For this review, take the finished solid that the model builds, in its own axes (mm). Face numbers are marked on the shaded views. A direction names the side the tool comes from. Coordinates: 2 decimals unless noted, no trailing zeros. Loops run counter-clockwise (first coordinate to the right, second up) from the corner with the lowest first, then second, coordinate; pieces in that order, holes last. Notation, with made-up numbers: (-15.5, 24) - (-11.5, 24) arc R26 ccw to (-11.5, 42) - close; hole circle Ø3 at (-4.75, 76.25). An arc over 180 degrees is marked (long way). Answer as a JSON object with one key per item and string values. Group by question number.
Item 1: Tool access review of the marked faces 1, 2, 3, 4 and 5: name each direction out of +Z, -Z, +X, -X, +Y, -Y from which nothing blocks a thin tool from reaching the whole face with its end or side.
Item 2: To check wall thickness, follow line 1 (Y direction, x = 10, z = 1.5); line 2 (Y direction, x = 63.5, z = 29); line 3 (Z direction, x = 60, y = 116.5). State the ranges of each line that lie inside material, in increasing order.
Item 3: We need section B-B (x = 38.5). State how many separate pieces and enclosed holes the cut face has, then the cut area to 3 significant figures.
Item 4: Clearance check with flat-ended pins moving along their axes: pin 1 (22.5 mm diameter, centred on x = 38, z = 18, fed in from -Y); pin 2 (3 mm diameter, centred on x = 44.5, y = 155, fed in from -Z); pin 3 (17.5 mm diameter, centred on x = 43, z = -4, fed in from +Y). State where each tip first meets the part, or that it passes through.
Item 5: We need section C-C (z = 24). Give the boundary of the cut face in (x, y), then the cut area to 3 significant figures.
Item 6: Mouldability with a two-part tool opening along Z and no side actions: class the marked faces 6, 7, 8 and 9 as released by +Z, released by -Z, zero draft, split by the parting line, or undercut.
Item 7: We need section A-A (z = 98). Give the boundary of the cut face in (x, y), then the cut area to 3 significant figures.
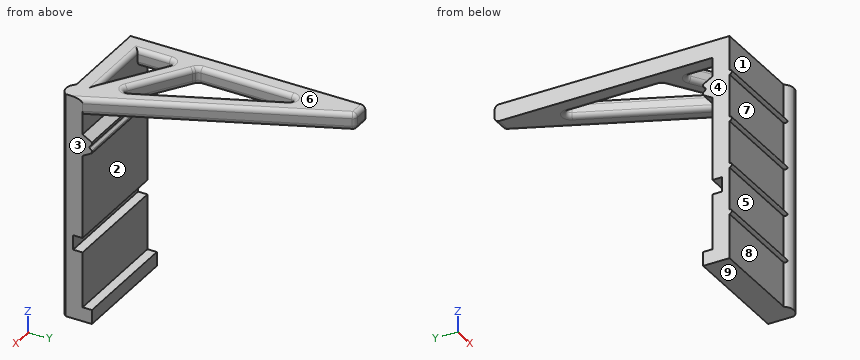
from build123d import *

# Parameters (mm, degrees)
EXTRUDE_1_DEPTH     = 120
SKETCH_2_W          = 15.5
SKETCH_2_H          = 10
CUT_EXTRUDE_1_DEPTH = 324.916484435
CUT_EXTRUDE_2_DEPTH = 40
CUT_EXTRUDE_3_DEPTH = 40
FILLET_16_R         = 5
EXTRUDE_2_DEPTH     = 239
EXTRUDE_3_DEPTH     = 18
FILLET_17_R         = 5
EXTRUDE_4_DEPTH     = 120
SKETCH_11_R         = 2.5
EXTRUDE_5_DEPTH     = 110
SKETCH_12_R         = 2.5
CUT_EXTRUDE_4_DEPTH = 324.916484528
FILLET_19_R         = 1


with BuildPart() as part:
    # 草圖1 → 填料-伸長1 (new body)
    with BuildSketch(Plane(origin=(0, 0, 0), x_dir=(0, 0, -1), z_dir=(1, 0, 0))):
        Polygon((-179.666666667, 241.333333333), (-179.666666667, -8.666666667), (59.333333333, -8.666666667), (59.333333333, 9.333333333), (59.333333333, 19.333333333), (44.333333333, 19.333333333), (44.333333333, 9.333333333), (-161.666666667, 9.333333333), (-161.666666667, 241.333333333), align=None)
    extrude(amount=EXTRUDE_1_DEPTH)

    # 草圖2 → 除料-伸長1 (cut, through all)
    with BuildSketch(Plane(origin=(120, 0, 0), x_dir=(0, 0, -1), z_dir=(1, 0, 0))):
        with Locations((-22.416666667, 4.333333333)):
            Rectangle(SKETCH_2_W, SKETCH_2_H)
    extrude(amount=-CUT_EXTRUDE_1_DEPTH, mode=Mode.SUBTRACT)

    # 草圖4 → 除料-伸長2 (cut)
    with BuildSketch(Plane.XY.offset(179.666666667)):
        Polygon((120, 241.333333333), (18, 241.333333333), (120, 9.333333333), align=None)
    extrude(amount=-CUT_EXTRUDE_2_DEPTH, mode=Mode.SUBTRACT)

    # 草圖5 → 除料-伸長3 (cut)
    with BuildSketch(Plane.XY.offset(179.666666667)):
        Polygon((100.337138528, 9.333333333), (18, 196.609962141), (18, 9.333333333), align=None)
    extrude(amount=-CUT_EXTRUDE_3_DEPTH, mode=Mode.SUBTRACT)

    # 圓角16
    # the kernel refuses this fillet: 5 mm, written as the material it takes off along each edge
    with BuildSketch(Plane(origin=(14.736369898, 236.333333333, 166.666666667), x_dir=(0, 1, 0), z_dir=(0, 0, -1))) as fillet_16_piece_1_section:
        Polygon((0, 0), (FILLET_16_R, 0), (FILLET_16_R, FILLET_16_R * 0.652726020499), (FILLET_16_R * 0.402474131984, FILLET_16_R * 0.915431359023), align=None)
    fillet_16_piece_1 = extrude(amount=FILLET_16_R, mode=Mode.PRIVATE)
    fillet_16_piece_1 = fillet_16_piece_1 - Plane(origin=(14.736369898, 236.333333333, 166.666666667), x_dir=(-0.5465921093537591, -0.8373989885306815, 0), z_dir=(0, 0, -1)) * Sphere(FILLET_16_R, mode=Mode.PRIVATE)
    add(fillet_16_piece_1, mode=Mode.SUBTRACT)
    with BuildSketch(Plane(origin=(14.736369898, 236.333333333, 174.666666667), x_dir=(0, 1, 0), z_dir=(0, 0, 1))) as fillet_16_piece_2_section:
        Polygon((0, 0), (FILLET_16_R, 0), (FILLET_16_R, -FILLET_16_R * 0.652726020499), (FILLET_16_R * 0.402474131984, -FILLET_16_R * 0.915431359023), align=None)
    fillet_16_piece_2 = extrude(amount=FILLET_16_R, mode=Mode.PRIVATE)
    fillet_16_piece_2 = fillet_16_piece_2 - Plane(origin=(14.736369898, 236.333333333, 174.666666667), x_dir=(-0.5465921093537591, -0.8373989885306815, 0), z_dir=(0, 0, 1)) * Sphere(FILLET_16_R, mode=Mode.PRIVATE)
    add(fillet_16_piece_2, mode=Mode.SUBTRACT)
    with BuildSketch(Plane(origin=(-12.5, 241.333333333, 161.666666667), x_dir=(0, 0, 1), z_dir=(1, 0, 0)), Plane(origin=(-12.5, 241.333333333, 179.666666667), x_dir=(0, -1, 0), z_dir=(1, 0, 0))) as fillet_16_piece_3:
        with BuildLine():
            CenterArc((FILLET_16_R, FILLET_16_R), FILLET_16_R, 180, 90)
            Line((0, FILLET_16_R), (0, 0))
            Line((0, 0), (FILLET_16_R, 0))
        make_face()
    extrude(amount=27.236369898, mode=Mode.SUBTRACT)
    with BuildSketch(Plane(origin=(18, 241.333333333, 174.666666667), x_dir=(-1, 0, 0), z_dir=(0, 0, -1))) as fillet_16_piece_4:
        with BuildLine():
            CenterArc((FILLET_16_R * 0.652726020499, -FILLET_16_R), FILLET_16_R, 90, 66.267060196)
            Line((-FILLET_16_R * 0.262705338524, -FILLET_16_R * 0.597525868016), (0, 0))
            Line((0, 0), (FILLET_16_R * 0.652726020499, 0))
        make_face()
    extrude(amount=8, mode=Mode.SUBTRACT)
    with BuildSketch(Plane(origin=(19.313526693, 238.345703993, 161.666666667), x_dir=(0, 0, 1), z_dir=(0.40247413198441667, -0.9154313590233789, 0))) as fillet_16_piece_5_section:
        with BuildLine():
            CenterArc((FILLET_16_R, FILLET_16_R), FILLET_16_R, 180, 90)
            Line((0, FILLET_16_R), (0, 0))
            Line((0, 0), (FILLET_16_R, 0))
        make_face()
    fillet_16_piece_5 = extrude(amount=262.668806653, mode=Mode.PRIVATE)
    fillet_16_piece_5 = split(fillet_16_piece_5, bisect_by=Plane(origin=(68.522420019, 9.333333333, 162.799850977), z_dir=(0, 1, 0)), keep=Keep.TOP, mode=Mode.PRIVATE)
    add(fillet_16_piece_5, mode=Mode.SUBTRACT)
    with BuildSketch(Plane(origin=(19.313526693, 238.345703993, 179.666666667), x_dir=(-0.9154313590233789, -0.40247413198441667, 5.6843418860808026e-15), z_dir=(0.40247413198441667, -0.9154313590233789, 0))) as fillet_16_piece_6:
        with BuildLine():
            CenterArc((FILLET_16_R, FILLET_16_R), FILLET_16_R, 180, 90)
            Line((0, FILLET_16_R), (0, 0))
            Line((0, 0), (FILLET_16_R, 0))
        make_face()
    extrude(amount=262.668806653, mode=Mode.SUBTRACT)

    # 草圖8 → 填料-伸長2 (add)
    with BuildSketch(Plane.XY.offset(179.666666667)):
        with BuildLine():
            ThreePointArc((110.17, -13.666666712), (115.684274668, -12.344840676), (120, -8.666666667))
            Line((120, -8.666666667), (110.17, -8.666666667))
            Line((110.17, -8.666666667), (110.17, -13.666666667))
        make_face()
        with BuildLine():
            Line((110.17, -13.666666667), (110.17, -8.666666667))
            Line((110.17, -8.666666667), (100.34, -8.666666667))
            ThreePointArc((100.34, -8.666666667), (104.655725332, -12.344840676), (110.17, -13.666666712))
        make_face()
        with BuildLine():
            ThreePointArc((110.17, -13.666666712), (115.684274668, -12.344840676), (120, -8.666666667))
            Line((120, -8.666666667), (110.17, -8.666666667))
            Line((110.17, -8.666666667), (110.17, -13.666666667))
        make_face()
        with BuildLine():
            Line((110.17, -13.666666667), (110.17, -8.666666667))
            Line((110.17, -8.666666667), (100.34, -8.666666667))
            ThreePointArc((100.34, -8.666666667), (104.655725332, -12.344840676), (110.17, -13.666666712))
        make_face()
    extrude(amount=-EXTRUDE_2_DEPTH)

    # 草圖9 → 填料-伸長3 (add)
    with BuildSketch(Plane.XY.offset(179.666666667)):
        Polygon((18, 63.079938443), (100.337138528, 9.333333333), (93.709875708, 24.407107589), (22.919522331, 70.616403134), (18, 73.827683351), align=None)
        Polygon((18, 52.332193536), (83.872125352, 9.333333333), (100.337138528, 9.333333333), (18, 63.079938443), align=None)
        Polygon((100.337138528, 9.333333333), (83.872125352, 9.333333333), (95.417616197, 1.796868643), align=None)
        Polygon((93.711170014, 24.406262715), (100.337138528, 9.333333333), (105.256660859, 16.869798024), align=None)
        Polygon((10.463535309, 67.999460774), (18, 63.079938443), (18, 73.827683351), (15.38305764, 75.535925465), align=None)
        Polygon((13.080477669, 55.543473753), (18, 52.332193536), (18, 63.079938443), align=None)
    extrude(amount=-EXTRUDE_3_DEPTH)

    # 圓角17
    fillet_17_edges = [part.edges().sort_by_distance(p)[0] for p in [
        (93.709875708, 24.407107589, 170.666666667),
        (18, 30.832763435, 179.666666667),
        (18, 30.832763435, 161.666666667),
        (18, 52.332193536, 170.666666667),
        (50.936062676, 30.832763435, 161.666666667),
        (50.936062676, 30.832763435, 179.666666667),
        (18, 73.827683351, 170.666666667),
        (55.854937854, 49.11739547, 179.666666667),
        (55.854937854, 49.11739547, 161.666666667),
        (55.854937854, 110.508534865, 161.666666667),
        (18, 135.218822746, 161.666666667),
        (18, 196.609962141, 170.666666667),
        (55.854937854, 110.508534865, 179.666666667),
        (18, 135.218822746, 179.666666667),
        (50.936062676, 9.333333333, 179.666666667),
    ]]
    fillet(fillet_17_edges, radius=FILLET_17_R)

    # 草圖10 → 填料-伸長4 (add)
    with BuildSketch(Plane(origin=(120, 0, 0), x_dir=(0, 0, -1), z_dir=(1, 0, 0))):
        Polygon((-118.619661283, 9.333333333), (-124.393163975, 19.333333333), (-135.940169359, 19.333333333), (-141.71367205, 9.333333333), (-135.940169359, -0.666666667), (-124.393163975, -0.666666667), align=None)
    extrude(amount=-EXTRUDE_4_DEPTH)

    # 草圖11 → 填料-伸長5 (add)
    with BuildSketch(Plane.ZY):
        with Locations((140.666666667, -8.666666667)):
            Circle(SKETCH_11_R)
        with Locations((90.666666667, -8.666666667)):
            Circle(SKETCH_11_R)
        with Locations((40.666666667, -8.666666667)):
            Circle(SKETCH_11_R)
        with Locations((-9.333333333, -8.666666667)):
            Circle(SKETCH_11_R)
    extrude(amount=-EXTRUDE_5_DEPTH)

    # 草圖12 → 除料-伸長4 (cut, through all)
    with BuildSketch(Plane(origin=(120, 0, 0), x_dir=(0, 0, -1), z_dir=(1, 0, 0))):
        with Locations((-130.168163975, 19.333333333)):
            Circle(SKETCH_12_R)
    extrude(amount=-CUT_EXTRUDE_4_DEPTH, mode=Mode.SUBTRACT)

    # 圓角19
    fillet_19_edges = [part.edges().sort_by_distance(p)[0] for p in [
        (60, 19.333333333, 127.668163975),
        (60, 19.333333333, 132.668163975),
    ]]
    fillet(fillet_19_edges, radius=FILLET_19_R)


solid = part.part
Check sheet entries:
{
 "1": {"face 1": "+Z, -X, -Y", "face 2": "+X, -X, +Y", "face 3": "+Z, -Z, +X, +Y, -Y", "face 4": "+Z, -Z, -X, +Y, -Y", "face 5": "-X, -Y"},
 "2": {"line 1": "y = -8.67 to 9.33", "line 2": "y = -8.67 to -0.67", "line 3": "z = 161.67 to 179.67"},
 "3": {"separate pieces": "3", "enclosed holes": "0", "area": "5,610 mm2"},
 "4": {"pin 1": "stops at y = -8.67", "pin 2": "stops at z = 161.67", "pin 3": "stops at y = 9.33"},
 "5": {"outline": "(0, -8.67) - (100.34, -8.67) arc R12.16 ccw to (120, -8.67) - (120, -0.67) - (0, -0.67) - close", "area": "1,030 mm2"},
 "6": {"face 6": "released by +Z", "face 7": "undercut", "face 8": "zero draft", "face 9": "released by -Z"},
 "7": {"outline": "(0, -8.67) - (100.34, -8.67) arc R12.16 ccw to (120, -8.67) - (120, 9.33) - (0, 9.33) - close", "area": "2,230 mm2"}
}
